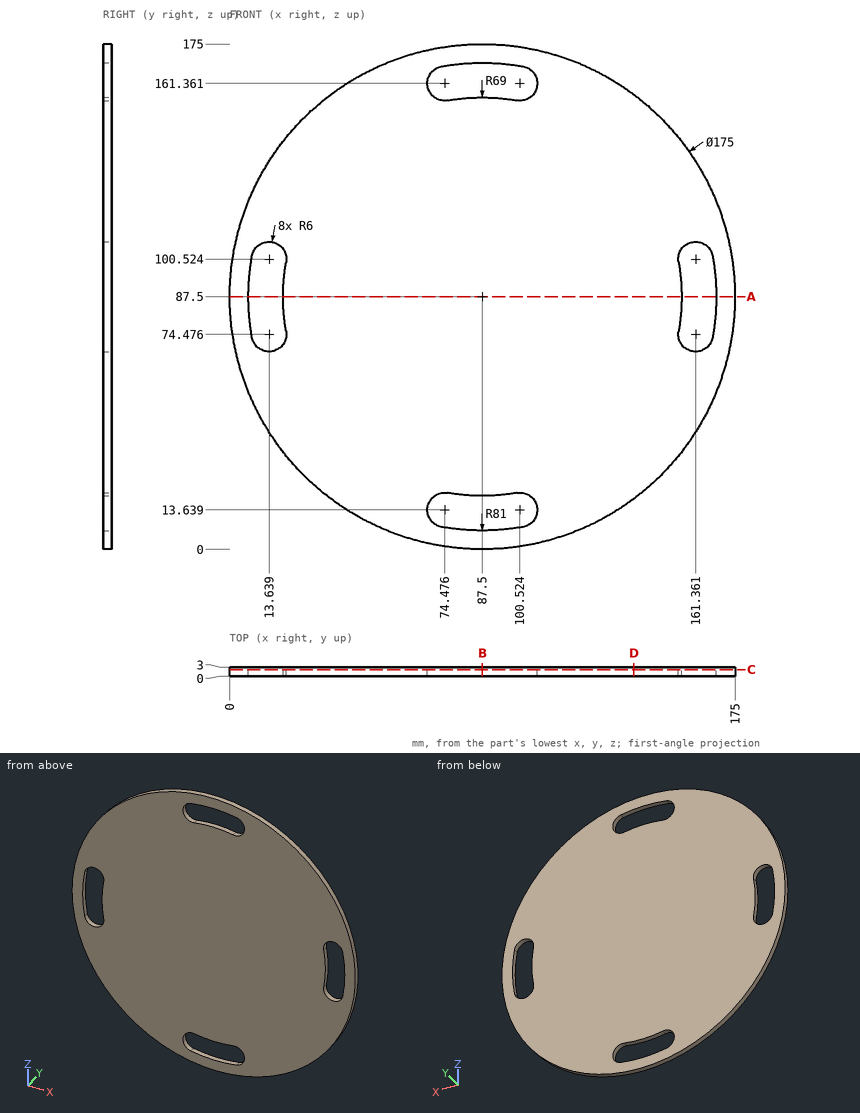
Print and shaded views of the part. All mm, measured from the part's lowest x, y and z. Give positions to 0.01 mm unless a question says otherwise; leave off trailing zeros. Loops run counter-clockwise (first coordinate to the right, second up) from the corner with the lowest first, then second, coordinate; pieces in that order, holes last. Notation, with made-up numbers: (63.25, 25.5) - (105.25, 25.5) arc R14 ccw to (105.25, 51.5) - close; hole circle Ø6 at (66.5, 75). An arc over 180 degrees is marked (long way). Use a Markdown table: item, result.
(1) Band-saw the part on B-B (x = 87.5). Give the cut face in (y, z).
Taken from the geometry:
| item | result |
|---|---|
| outline | (0, 0) - (3, 0) - (3, 6.5) - (0, 6.5) - close; (0, 18.5) - (3, 18.5) - (3, 156.5) - (0, 156.5) - close; (0, 168.5) - (3, 168.5) - (3, 175) - (0, 175) - close |
(2) Wall check: line 1 along Z through (x, y) = (86.5, 1.6) (1 decimal); line 2 along X through (y, z) = (1.15, 74). Give the ranges that are in metal, low to high.
Taken from the geometry:
| item | result |
|---|---|
| line 1 | 0 to 6.5, 18.5 to 156.5, 168.5 to 175 |
| line 2 | 1.05 to 7.63, 19.62 to 155.38, 167.37 to 173.95 |
(3) Band-saw the part on A-A (z = 87.5). Give the cut face in (x, y), and give its area (3 significant figures).
Taken from the geometry:
| item | result |
|---|---|
| outline | (0, 0) - (6.5, 0) - (6.5, 3) - (0, 3) - close; (18.5, 0) - (156.5, 0) - (156.5, 3) - (18.5, 3) - close; (168.5, 0) - (175, 0) - (175, 3) - (168.5, 3) - close |
| area | 453 mm2 |
(4) Band-saw the part on C-C (y = 2.25). Give the cut face in (x, z) (1 decimal), and give its area (3 significant figures).
Taken from the geometry:
| item | result |
|---|---|
| outline | circle Ø175 at (87.5, 87.5); hole (7.7, 73.4) arc R6 ccw to (19.5, 75.5) arc R69 cw to (19.5, 99.5) arc R6 ccw to (7.7, 101.6) arc R81 ccw to start; hole (73.4, 7.7) arc R81 ccw to (101.6, 7.7) arc R6 ccw to (99.5, 19.5) arc R69 cw to (75.5, 19.5) arc R6 ccw to start; hole (73.4, 167.3) arc R6 ccw to (75.5, 155.5) arc R69 cw to (99.5, 155.5) arc R6 ccw to (101.6, 167.3) arc R81 ccw to start; hole (155.5, 75.5) arc R6 ccw to (167.3, 73.4) arc R81 ccw to (167.3, 101.6) arc R6 ccw to (155.5, 99.5) arc R69 cw to start |
| area | 22,300 mm2 |
(5) Band-saw the part on D-D (x = 140). Give the cut face in (y, z).
Taken from the geometry:
| item | result |
|---|---|
| outline | (0, 17.5) - (3, 17.5) - (3, 157.5) - (0, 157.5) - close |
